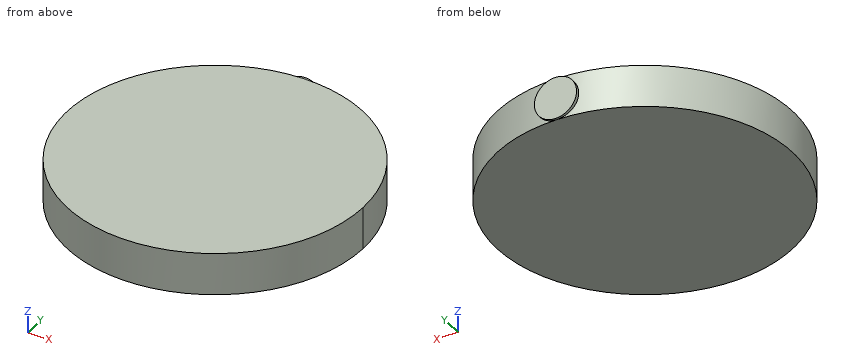
Autodesk Inventor part; units mm, degrees
ref_plane "YZ Plane" through (0, 0, 0) normal (1, 0, 0) x (0, 1, 0)
ref_plane "XZ Plane" through (0, 0, 0) normal (0, 1, 0) x (-1, 0, 0)
ref_plane "XY Plane" through (0, 0, 0) normal (0, 0, 1) x (1, 0, 0)
sketch "Эскиз3" plane through (0, 0, 0) normal (0, 0, 1) x (1, 0, 0)
  circle A0 centre (0, 0) radius 70
  dimension "d1" = 140
extrude "Выдавливание1" add sketch "Эскиз3" along normal mid plane 20
sketch "Эскиз4" plane through (0, 0, 0) normal (0, 1, 0) x (-1, 0, 0)
  circle A0 centre (0, 0) radius 10
  dimension "d4" = 20
extrude "Выдавливание2" add sketch "Эскиз4" along normal blind 71
equation "\"d1\" = hip_diam"
equation "\"d4\" = joint_width"
properties part number "ч ASY human dummy 01"
Design review of the part built by this model. Coordinates are the model's own, in mm. Coordinates: 2 decimals unless noted, no trailing zeros. Write each loop counter-clockwise with the first axis right and the second up, starting at its lowest first coordinate (ties: lowest second). Pieces come first, ordered by that corner, then holes. Notation, with made-up numbers: (26.25, 34) -> (56.25, 34) arc R12 ccw to (56.25, 48) -> close; hole circle Ø8 at (70.25, -27.5). An arc over 180 degrees is marked (long way). Write each question's results on one line, items separated by ' | '. Start each with the question number.
(1) For line 1 along Y through (x, z) = (-1, 7.25); line 2 along X through (y, z) = (57, 0.5); line 3 along X through (y, z) = (-60.5, 7.5), list the stretches that pass through material, from the lowest coordinate up. Write a range as from..to.
(2) Clearance check with flat-ended pins moving along their axes: P1, Ø4, axis at y = -24.5, z = -0.5, coming from the +X side; P2, Ø1.5, axis at y = 23.5, z = 2, coming from the -X side; P3, Ø6, axis at x = -2, z = 2, coming from the -Y side. State where each tip first meets the part, or that it passes through.
(3) Take a section at A-A on z = 0. Write out the cut boundary in (x, y).
(4) Take a section at B-B on x = -53. Write out the cut boundary in (y, z), and give its area (3 significant figures).
Results found:
1) line 1: y = -69.99..71 | line 2: x = -40.63..40.63 | line 3: x = -35.21..35.21
2) P1: stops at x = 66.29 | P2: stops at x = -66.2 | P3: stops at y = -70
3) outline: (-10, 69.28) arc R70 ccw (long way) to (10, 69.28) -> (10, 71) -> (-10, 71) -> close
4) outline: (-45.73, -10) -> (45.73, -10) -> (45.73, 10) -> (-45.73, 10) -> close | area: 1,830 mm2
